Part print with two shaded views. Sizes in mm from the minimum x, y, z corner. A direction names the side the tool comes from. Round coordinates to 2 decimals unless told otherwise and drop trailing zeros. Write each loop counter-clockwise with the first axis right and the second up, starting at its lowest first coordinate (ties: lowest second). Pieces come first, ordered by that corner, then holes. Notation, with made-up numbers: (83, -11) -> (106, -11) arc R24 cw to (106, 2) -> close; hole circle Ø4 at (84, 21). An arc over 180 degrees is marked (long way). Return JSON: item names as keys, results as strings.
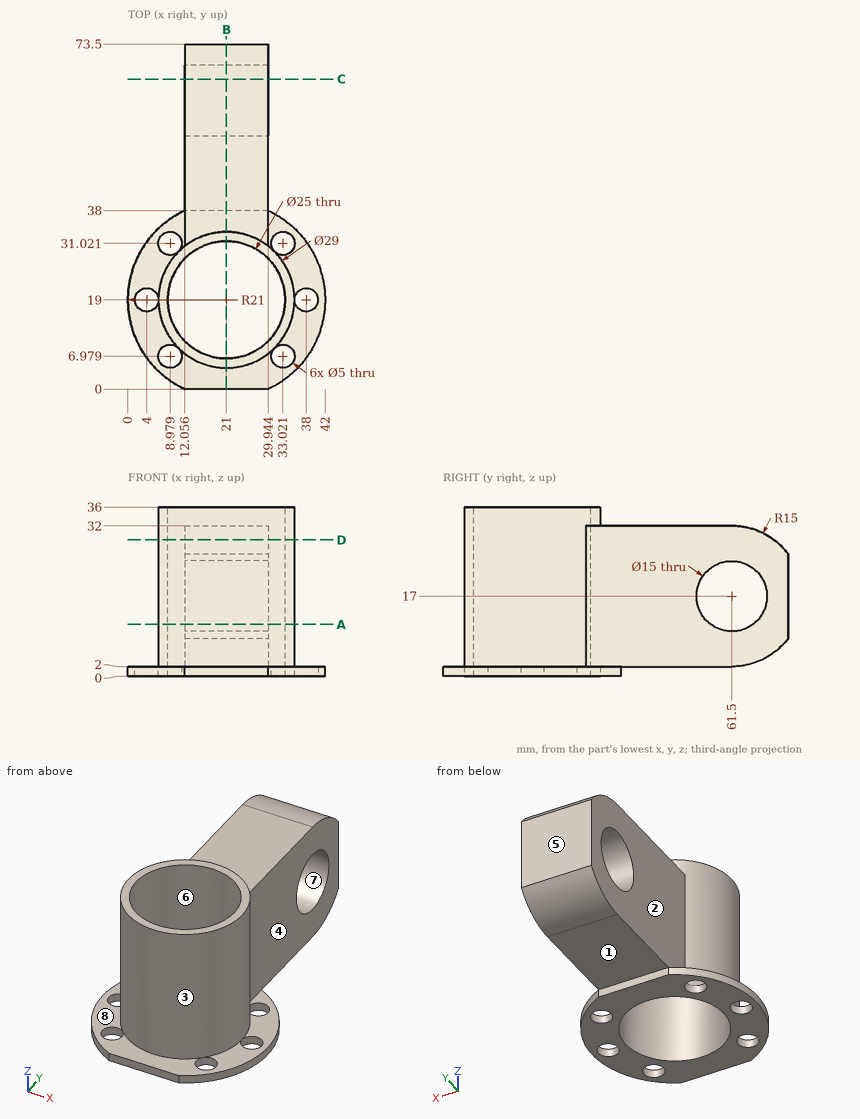
Q1. Saw through at B-B on x = 21. List the corners of the cut face in (y, z).
Verdict:
{"outline": "(0, 0) -> (6.5, 0) -> (6.5, 36) -> (4.5, 36) -> (4.5, 2) -> (0, 2) -> close; (31.5, 0) -> (38, 0) -> (38, 2) -> (61.5, 2) arc R15 ccw to (73.5, 8) -> (73.5, 26) arc R15 ccw to (61.5, 32) -> (33.5, 32) -> (33.5, 36) -> (31.5, 36) -> close; hole circle Ø15 at (61.5, 17)"}
Q2. Wall check: L1, parallel to Y at x = 22, z = 18 (1 decimal); L2, parallel to X at y = 19.5, z = 10.5; L3, parallel to X at y = 48, z = 27. Give the ranges that are in metal, low to high.
Verdict:
{"L1": "y = 4.5 to 6.5, 31.5 to 54.1, 68.9 to 73.5", "L2": "x = 6.51 to 8.51, 33.49 to 35.49", "L3": "x = 12.06 to 29.94"}
Q3. Saw through at A-A on z = 11. List the corners of the cut face in (x, y).
Verdict:
{"outline": "(12.06, 30.41) arc R14.5 ccw (long way) to (29.94, 30.41) -> (29.94, 57) -> (12.06, 57) -> close; (12.06, 66) -> (29.94, 66) -> (29.94, 73.5) -> (12.06, 73.5) -> close; hole circle Ø25 at (21, 19)"}
Q4. Pin check, flat tips, straight feed: pin 1 Ø3 at (x, y) = (8.98, 31.02) entering from -Z; pin 2 Ø15 at (y, z) = (42.5, 20) entering from -X; pin 3 Ø4 at (x, y) = (30, 53) entering from -Z; pin 4 Ø9 at (x, y) = (20, 40.5) entering from +Z. Stop position of each tip, or through.
Verdict:
{"pin 1": "passes through", "pin 2": "stops at x = 12.06", "pin 3": "stops at z = 2", "pin 4": "stops at z = 32"}
Q5. Saw through at C-C on y = 66. List the corners of the cut face in (x, z).
Verdict:
{"outline": "(12.06, 2.69) -> (29.94, 2.69) -> (29.94, 11) -> (12.06, 11) -> close; (12.06, 23) -> (29.94, 23) -> (29.94, 31.31) -> (12.06, 31.31) -> close"}
Q6. 3-axis set-ups, long thin cutter, end or side, ignore diameter. For the marked faces 1, 2, 3, 4 and 5: which of +Z, -Z, +X, -X, +Y, -Y reach the whole face in a straight line?
Verdict:
{"face 1": "-Z, +X, -X, +Y", "face 2": "+Z, -X, +Y", "face 3": "+Z", "face 4": "+Z, +X, +Y", "face 5": "+Z, -Z, +X, -X, +Y"}
Q7. Two-plate mould, pull along Z, no slides. Class the marked faces 6, 7 and 8: +Z half, -Z half, draft (parallel to the pull), parting line (faces both ways), or undercut.
Verdict:
{"face 6": "draft", "face 7": "undercut", "face 8": "+Z half"}
Q8. Saw through at D-D on z = 29. List the corners of the cut face in (x, y).
Verdict:
{"outline": "(12.06, 30.41) arc R14.5 ccw (long way) to (29.94, 30.41) -> (29.94, 70.5) -> (12.06, 70.5) -> close; hole circle Ø25 at (21, 19)"}
